from build123d import *

# Parameters (mm, degrees)
SKETCH_W              = 150
SKETCH_H              = 25
PAD_DEPTH             = 3
PAD001_DEPTH          = 3
SKETCH004_W           = 150
SKETCH004_H           = 25
SKETCH004_W_2         = 96
SKETCH004_H_2         = 2.8
PAD002_DEPTH          = 3
SKETCH005_R           = 0.85
POCKET_DEPTH          = 313.671314
POLARPATTERN_COUNT    = 2
POLARPATTERN001_COUNT = 2
POLARPATTERN002_COUNT = 2
FILLET_R              = 5


with BuildPart() as part:
    # Sketch → Pad (new body)
    with BuildSketch(Plane.XY):
        Rectangle(SKETCH_W, SKETCH_H)
    extrude(amount=PAD_DEPTH)

    # Sketch001 (on Face6 of Pad) → Pad001 (join)
    with BuildSketch(Plane.XY.offset(3)):
        Polygon((-75, 12.5), (75, 12.5), (75, 4), (50, 4), (50, 5), (-50, 5), (-50, 4), (-52.25, 4), (-52.25, 9.2), (-72.25, 9.2), (-72.25, 4.5), (-75, 4.5), align=None)
        Polygon((-75, -12.5), (75, -12.5), (75, -4), (50, -4), (50, -5), (-50, -5), (-50, -4), (-52.25, -4), (-52.25, -9.2), (-72.25, -9.2), (-72.25, -4.5), (-75, -4.5), align=None)
    extrude(amount=PAD001_DEPTH)

    # Sketch004 (on Face12 of Pad001) → Pad002 (join)
    with BuildSketch(Plane.XY.offset(6)):
        Rectangle(SKETCH004_W, SKETCH004_H)
        Rectangle(SKETCH004_W_2, SKETCH004_H_2, mode=Mode.SUBTRACT)
    extrude(amount=PAD002_DEPTH)

    # Sketch005 (on Face34 of Pad002) → Pocket (cut, through all)
    with BuildSketch(Plane.XY.offset(9)):
        with Locations((-70, 7.5)):
            Circle(SKETCH005_R)
    pocket = extrude(amount=-POCKET_DEPTH, mode=Mode.SUBTRACT)

    # PolarPattern: Pocket ×2 about axis
    polarpattern_axis = Axis((0, 0, 9), (0, 0, 1))
    for i in range(1, POLARPATTERN_COUNT):
        add(pocket.rotate(polarpattern_axis, i * 360 / POLARPATTERN_COUNT), mode=Mode.SUBTRACT)

    # PolarPattern001: Pocket ×2 about axis
    polarpattern001_axis = Axis((0, 0, 0), (0, 1, 0))
    for i in range(1, POLARPATTERN001_COUNT):
        add(pocket.rotate(polarpattern001_axis, i * 360 / POLARPATTERN001_COUNT), mode=Mode.SUBTRACT)

    # PolarPattern002: Pocket ×2 about axis
    polarpattern002_axis = Axis((0, 0, 0), (1, 0, 0))
    for i in range(1, POLARPATTERN002_COUNT):
        add(pocket.rotate(polarpattern002_axis, i * 360 / POLARPATTERN002_COUNT), mode=Mode.SUBTRACT)

    # Fillet
    fillet_edges = [part.edges().sort_by_distance(p)[0] for p in [
        (75, -12.5, 7.5),
        (75, 12.5, 7.5),
        (-75, -12.5, 7.5),
        (-75, 12.5, 7.5),
    ]]
    fillet(fillet_edges, radius=FILLET_R)


solid = part.part
Model file for the job. Use its own axes, mm. A direction names the side the tool comes from. Give positions to 0.01 mm unless a question says otherwise; leave off trailing zeros. Loops run counter-clockwise (first coordinate to the right, second up) from the corner with the lowest first, then second, coordinate; pieces in that order, holes last. Notation, with made-up numbers: (50.25, 86) - (75.25, 86) arc R32 cw to (75.25, 113) - close; hole circle Ø7 at (74.5, -6). An arc over 180 degrees is marked (long way). Use one line per item in the form item = value.
(1) Drop flat-ended pins along their axis: P1, Ø3, axis at x = -74.5, z = 5, coming from the +Y side; P2, Ø2.5, axis at x = 70, y = -7.5, coming from the +Z side; P3, Ø0.8, axis at x = -73.5, z = 4, coming from the -Y side. Give the stop position or say it passes through.
Determined:
P1 = 11.5
P2 = 9
P3 = -11.42
(2) Cut at B-B (x = -63.5). Give the cut face in (y, z).
Determined:
outline = (-12.5, 0) - (12.5, 0) - (12.5, 9) - (-12.5, 9) - close; hole (-9.2, 3) - (9.2, 3) - (9.2, 6) - (-9.2, 6) - close
(3) Pull direction Y, two halves, no side cores. Call faces 1 (the face through (-1, 12.5, 4)), 2 (the face through (-72.25, -7, 4)), 3 (the face through (-1, 0, 0)): pulls with the +Y half, pulls with the -Y half, needs draft (parallel to the pull), parting line crosses it, or undercut.
Determined:
face_1 = pulls with the +Y half
face_2 = undercut
face_3 = needs draft
(4) Cut at A-A (y = 2.75). Give the cut face in (x, z).
Determined:
outline = (-75, 0) - (75, 0) - (75, 3) - (-75, 3) - close; (-75, 6) - (75, 6) - (75, 9) - (-75, 9) - close
(5) Cut at C-C (x = 4). Give the cut face in (y, z).
Determined:
outline = (-12.5, 0) - (12.5, 0) - (12.5, 9) - (1.4, 9) - (1.4, 6) - (5, 6) - (5, 3) - (-5, 3) - (-5, 6) - (-1.4, 6) - (-1.4, 9) - (-12.5, 9) - close
(6) 3-axis set-ups, long thin cutter, end or side, ignore diameter. For faces 4 (the face through (-1, -2, 6)), 5 (the face through (63, -4, 4)), 6 (the face through (48, 0, 7)), 7 (the face through (-74, 4.5, 4)): which of +Z, -Z, +X, -X, +Y, -Y reach the whole face in a straight line?
Determined:
face_4 = none
face_5 = +X, -X
face_6 = +Z
face_7 = -X
(7) Drill centre lines: L1, parallel to Y at x = -70, z = 7.4; L2, parallel to X at y = -7.5, z = 0.7; L3, parallel to Y at x = 58.5, z = 4.5. Where is each one in solid material? Low to high.
Determined:
L1 = -12.5 to -8.35, -6.65 to 6.65, 8.35 to 12.5
L2 = -75 to -70.85, -69.15 to 69.15, 70.85 to 75
L3 = -12.5 to -4, 4 to 12.5
